Autodesk Inventor part; units mm, degrees
ref_plane "YZ Plane" through (0, 0, 0) normal (1, 0, 0) x (0, 1, 0)
ref_plane "XZ Plane" through (0, 0, 0) normal (0, 1, 0) x (-1, 0, 0)
ref_plane "XY Plane" through (0, 0, 0) normal (0, 0, 1) x (1, 0, 0)
sketch "Boceto1" plane through (0, 0, 0) normal (0, 1, 0) x (-1, 0, 0)
  circle A0 centre (0, 0) radius 14.4
  circle A1 centre (0, 0) radius 15.9
  dimension "d0" = 28.8
  dimension "d1" = 1.5
extrude "Extrusión1" add sketch "Boceto1" along normal blind 22
sketch "Boceto2" plane through (0, 0, 0) normal (0, 0, 1) x (1, 0, 0)
  line L0 (15.9, 22) -> (-15.9, 22)
  point P0 (0, 0)
  point P1 (0, 7)
  dimension "d4" = 15
hole "Agujero1" at (0, 7, 0) direction (0, 0, -1) diameter 7 end through all
sketch "Boceto3" plane through (0, 22, 0) normal (0, 1, 0) x (1, 0, 0)
  circle A0 centre (0, 0) radius 15.9
  circle A1 centre (0, 0) radius 10
  dimension "d12" = 20
extrude "Extrusión2" add sketch "Boceto3" along normal blind 6
sketch "Boceto4" plane through (0, 28, 0) normal (0, 1, 0) x (1, 0, 0)
  circle A0 centre (0, 0) radius 15.9
  circle A1 centre (0, 0) radius 6
  dimension "d15" = 12
extrude "Extrusión3" add sketch "Boceto4" along normal blind 3
properties part number "limite_3DPrint"
Source: CAD feature listing. Evaluate the final solid. Frame: model axes, mm. A direction names the side the tool comes from. Coordinates: 2 decimals unless noted, no trailing zeros. Loops run counter-clockwise (first coordinate to the right, second up) from the corner with the lowest first, then second, coordinate; pieces in that order, holes last. Notation, with made-up numbers: (-19.5, 18.5) - (-1.5, 18.5) arc R20 ccw to (-1.5, 39.5) - close; hole circle Ø10 at (31, -30.5). An arc over 180 degrees is marked (long way). Answer as CSV lines item,"result".
1. Section A-A (x = 0). Return loops of the section in (y, z), then the cut area to 3 significant figures.
Established:
outline,"(0, -15.9) - (3.5, -15.9) - (3.5, -14.4) - (0, -14.4) - close; (0, 14.4) - (22, 14.4) - (22, 10) - (28, 10) - (28, 6) - (31, 6) - (31, 15.9) - (0, 15.9) - close; (10.5, -15.9) - (31, -15.9) - (31, -6) - (28, -6) - (28, -10) - (22, -10) - (22, -14.4) - (10.5, -14.4) - close"
area,"186 mm2"
2. Mould query, pull axis Z, two halves, no side actions, for faces 4 (the flat face through (4, 0, 14)), 5 (the flat face through (7, 28, 0)), 6 (the flat face through (-10, 22, 3)). Classes: released by +Z, released by -Z, zero draft, split by the parting line, or undercut.
Established:
face 4,"zero draft"
face 5,"undercut"
face 6,"undercut"
3. Section B-B (z = 0). Return loops of the section in (x, y).
Established:
outline,"(-15.9, 0) - (-14.4, 0) - (-14.4, 22) - (-10, 22) - (-10, 28) - (-6, 28) - (-6, 31) - (-15.9, 31) - close; (6, 28) - (10, 28) - (10, 22) - (14.4, 22) - (14.4, 0) - (15.9, 0) - (15.9, 31) - (6, 31) - close"
4. Reachability of faces 1 (the cylindrical face through (-6, 29, 0)), 2 (the cylindrical face through (-2.17, 24.96, -9.76)), 3 (the cylindrical face through (3.105, 5.385, -14.948)) from +Z, -Z, +X, -X, +Y, -Y: full face, straight path, thin tool, end or side. Return the list, or none.
Established:
face 1,"+Y, -Y"
face 2,"-Y"
face 3,"-Z"
5. Section D-D (x = -4). Return loops of the section in (y, z).
Established:
outline,"(0, -15.39) - (31, -15.39) - (31, -4.47) - (28, -4.47) - (28, -9.17) - (22, -9.17) - (22, -13.83) - (0, -13.83) - close; (0, 13.83) - (22, 13.83) - (22, 9.17) - (28, 9.17) - (28, 4.47) - (31, 4.47) - (31, 15.39) - (0, 15.39) - close"
6. Section C-C (y = 18). Return loops of the section in (x, z).
Established:
outline,"circle Ø31.8 at (0, 0); hole circle Ø28.8 at (0, 0)"
7. Contact query for flat-ended pins moving along their axis: pin 1 (6 mm diameter, centred on x = 1, z = -0.5, fed in from -Y); pin 2 (8 mm diameter, centred on x = 5, y = 15.5, fed in from -Z); pin 3 (1.5 mm diameter, centred on y = 19.5, z = -10, fed in from -X); pin 4 (1 mm diameter, centred on y = 16, z = 8, fed in from +X). Output: stop coordinate, or through.
Established:
pin 1,"passes through"
pin 2,"stops at z = -15.87"
pin 3,"stops at x = -12.93"
pin 4,"stops at x = 14.02"
8. Ray query, line 1 (Z direction, x = 0, y = 24.4); line 2 (Y direction, x = 0, z = -15.25). Return the intervals inside material, ascending.
Established:
line 1,"z = -15.9 to -10, 10 to 15.9"
line 2,"y = 0 to 3.5, 10.5 to 31"
